```python
from build123d import *

# Parameters (mm, degrees)
BOSS_EXTRUDE1_OUTLINE_R        = 14.5
BOSS_EXTRUDE1_DEPTH            = 3.175
M4_CLEARANCE_HOLE1_D           = 4.5
F_3_3_3_3_DIAMETER_HOLE4_D     = 3.3
M3_CLEARANCE_HOLE2_D           = 3.4
M2X0_4_TAPPED_HOLE2_AT_2_COUNT = 2
M2X0_4_TAPPED_HOLE2_AT_2_PITCH = 86
M2X0_4_TAPPED_HOLE2_AT_3_COUNT = 2
M2X0_4_TAPPED_HOLE2_AT_3_PITCH = 103.730419839
M2X0_4_TAPPED_HOLE2_AT_4_COUNT = 2
M2X0_4_TAPPED_HOLE2_AT_4_PITCH = 58
FILLET1_R                      = 3
FILLET2_R                      = 1
FILLET3_SIZE                   = 6
FILLET3_SIZE_2                 = 9
FILLET4_R                      = 5
M3_CLEARANCE_HOLE1_D           = 3.4
M3_CLEARANCE_HOLE1_CSINK_D     = 3.45
M3_CLEARANCE_HOLE1_CSINK_ANGLE = 90
M2X0_4_TAPPED_HOLE1_D          = 1.6


with BuildPart() as part:
    # Boss-Extrude1: read off the stored shape, not the designer's step
    # Boss-Extrude1 outline → Boss-Extrude1 (new body)
    with BuildSketch(Plane(origin=(0, 0, 0), x_dir=(1, 0, 0), z_dir=(0, 1, 0))):
        with BuildLine():
            Line((33, 11.630595388), (33, 78.33262411))
            ThreePointArc((33, 78.33262411), (28.545123253, 80.063574355), (24, 81.541400528))
            Line((24, 81.541400528), (24, 45))
            Line((24, 45), (13, 45))
            Line((13, 45), (13, 24))
            Line((13, 24), (-13, 24))
            Line((-13, 24), (-13, 45))
            Line((-13, 45), (-24, 45))
            Line((-24, 45), (-24, 81.541400528))
            ThreePointArc((-24, 81.541400528), (-28.545123253, 80.063574355), (-33, 78.33262411))
            Line((-33, 78.33262411), (-33, 11.630595388))
            Line((-33, 11.630595388), (-49.185297029, 11.630595388))
            Line((-49.185297029, 11.630595388), (-52.624325057, 21.384301413))
            Line((-52.624325057, 21.384301413), (-58.624325057, 21.384301413))
            Line((-58.624325057, 21.384301413), (-58.624325057, 26.630595388))
            Line((-58.624325057, 26.630595388), (-68.191318528, 26.630595388))
            Line((-68.191318528, 26.630595388), (-77.073860284, 35.841596796))
            ThreePointArc((-77.073860284, 35.841596796), (-84.367778143, 10.347850562), (-83.451078309, -16.152941807))
            Line((-83.451078309, -16.152941807), (-75.073268231, -10.906716078))
            Line((-75.073268231, -10.906716078), (-66.121429656, -10.906716078))
            Line((-66.121429656, -10.906716078), (-53.091566877, -24.906716078))
            Line((-53.091566877, -24.906716078), (-34.205297029, -24.906716078))
            Line((-34.205297029, -24.906716078), (-34.205297029, -39))
            Line((-34.205297029, -39), (60.196181169, -39))
            Line((60.196181169, -39), (60.196181169, -17.27312839))
            Line((60.196181169, -17.27312839), (66.121429656, -10.906716078))
            Line((66.121429656, -10.906716078), (75.073268231, -10.906716078))
            Line((75.073268231, -10.906716078), (83.451078309, -16.152941807))
            ThreePointArc((83.451078309, -16.152941807), (84.367778143, 10.347850562), (77.073860284, 35.841596796))
            Line((77.073860284, 35.841596796), (55.268726082, 28.884301413))
            Line((55.268726082, 28.884301413), (49.185297029, 11.630595388))
            Line((49.185297029, 11.630595388), (33, 11.630595388))
        make_face()
        with Locations((-68.685297029, 8.424)):
            Circle(BOSS_EXTRUDE1_OUTLINE_R, mode=Mode.SUBTRACT)
        Polygon((-49.185297029, -18.906716078), (-49.185297029, 7.630595388), (-29, 7.630595388), (-29, 20.630595388), (-21.3, 20.630595388), (-21.3, -18.906716078), align=None, mode=Mode.SUBTRACT)
        Polygon((29, 20.630595388), (29, 7.630595388), (49.185297029, 7.630595388), (49.185297029, -27.138060345), (21.3, -27.138060345), (21.3, 20.630595388), align=None, mode=Mode.SUBTRACT)
        with Locations((68.685297029, 8.424)):
            Circle(BOSS_EXTRUDE1_OUTLINE_R, mode=Mode.SUBTRACT)
    extrude(amount=BOSS_EXTRUDE1_DEPTH)

    # M4 Clearance Hole1 (through all)
    with Locations(Plane(origin=(0, 3.175, 0), x_dir=(1, 0, 0), z_dir=(0, 1, 0))):
        with Locations((-78.54120923, -8.5016735), (78.54120923, -8.5016735)):
            Hole(M4_CLEARANCE_HOLE1_D / 2)

    # Ø3.3 (3.3) Diameter Hole4 (through all)
    with Locations(Plane(origin=(0, 3.175, 0), x_dir=(1, 0, 0), z_dir=(0, 1, 0))):
        with Locations((17.5, 15.4), (-17.5, -18), (-17.5, 15.4), (17.5, -18)):
            Hole(F_3_3_3_3_DIAMETER_HOLE4_D / 2)

    # M3 Clearance Hole2 (through all)
    with Locations(Plane(origin=(0, 3.175, 0), x_dir=(1, 0, 0), z_dir=(0, 1, 0))):
        with Locations((28.19, 74.751400528), (-28.19, 74.751400528)):
            Hole(M3_CLEARANCE_HOLE2_D / 2)

    # Sketch15 → M2x0.4 Tapped Hole2 (revolve, cut)
    with BuildSketch(Plane(origin=(-29.558455866, 3.175, -25.380595388), x_dir=(0, 0, 1), z_dir=(1, 0, 0))):
        Polygon((0, 0), (0, 3.175), (1.5, 3.175), (0.8, 2.475), (0.8, 0), align=None)
    m2x0_4_tapped_hole2 = revolve(axis=Axis((-29.558455866, 9.525, -25.380595388), (0, -1, 0)), mode=Mode.SUBTRACT)

    # M2x0.4 Tapped Hole2 at 2: M2x0.4 Tapped Hole2 ×2
    with Locations(*[(i * M2X0_4_TAPPED_HOLE2_AT_2_PITCH, 0, 0) for i in range(1, M2X0_4_TAPPED_HOLE2_AT_2_COUNT)]):
        add(m2x0_4_tapped_hole2, mode=Mode.SUBTRACT)

    # M2x0.4 Tapped Hole2 at 3: M2x0.4 Tapped Hole2 ×2
    with Locations(*[Vector(0.8290721288256765, 0, 0.5591416682777818) * (i * M2X0_4_TAPPED_HOLE2_AT_3_PITCH) for i in range(1, M2X0_4_TAPPED_HOLE2_AT_3_COUNT)]):
        add(m2x0_4_tapped_hole2, mode=Mode.SUBTRACT)

    # M2x0.4 Tapped Hole2 at 4: M2x0.4 Tapped Hole2 ×2
    with Locations(*[(0, 0, i * M2X0_4_TAPPED_HOLE2_AT_4_PITCH) for i in range(1, M2X0_4_TAPPED_HOLE2_AT_4_COUNT)]):
        add(m2x0_4_tapped_hole2, mode=Mode.SUBTRACT)

    # Fillet1
    fillet1_edges = [part.edges().sort_by_distance(p)[0] for p in [
        (75.073268231, 1.5875, 10.906716078),
        (66.121429656, 1.5875, 10.906716078),
        (-66.121429656, 1.5875, 10.906716078),
        (-75.073268231, 1.5875, 10.906716078),
        (-68.191318528, 1.5875, -26.630595388),
        (-33, 1.5875, -78.33262411),
        (-24, 1.5875, -81.541400528),
        (24, 1.5875, -81.541400528),
        (33, 1.5875, -78.33262411),
    ]]
    fillet(fillet1_edges, radius=FILLET1_R)

    # Fillet2
    fillet2_edges = [part.edges().sort_by_distance(p)[0] for p in [
        (33, 1.5875, -11.630595388),
        (49.185297029, 1.5875, -11.630595388),
        (55.268726082, 1.5875, -28.884301413),
        (77.073860284, 1.5875, -35.841596796),
        (83.451078309, 1.5875, 16.152941807),
        (60.196181169, 1.5875, 17.27312839),
        (60.196181169, 1.5875, 39),
        (-34.205297029, 1.5875, 39),
        (-34.205297029, 1.5875, 24.906716078),
        (-53.091566877, 1.5875, 24.906716078),
        (-83.451078309, 1.5875, 16.152941807),
        (-77.073860284, 1.5875, -35.841596796),
        (-58.624325057, 1.5875, -26.630595388),
        (-58.624325057, 1.5875, -21.384301413),
        (-52.624325057, 1.5875, -21.384301413),
        (-49.185297029, 1.5875, -11.630595388),
        (-33, 1.5875, -11.630595388),
        (-24, 1.5875, -45),
        (-13, 1.5875, -45),
        (13, 1.5875, -45),
        (24, 1.5875, -45),
        (-49.185297029, 1.5875, -7.630595388),
        (-21.3, 1.5875, -20.630595388),
        (-29, 1.5875, -20.630595388),
        (-29, 1.5875, -7.630595388),
        (29, 1.5875, -20.630595388),
        (21.3, 1.5875, -20.630595388),
        (49.185297029, 1.5875, -7.630595388),
        (29, 1.5875, -7.630595388),
    ]]
    fillet(fillet2_edges, radius=FILLET2_R)

    # Fillet3
    # a fillet whose section is not a circle: 9, 6 mm, written as the material it adds along each edge
    with BuildSketch(Plane(origin=(13, 0, -24), x_dir=(0, 0, -1), z_dir=(0, 1, 0))) as fillet3_piece_1:
        with BuildLine():
            Bezier((FILLET3_SIZE, 0), (0, 0), (0, FILLET3_SIZE_2), weights=[1, 0.666666667, 1])
            Line((0, FILLET3_SIZE_2), (0, 0))
            Line((0, 0), (FILLET3_SIZE, 0))
        make_face()
    extrude(amount=3.175)
    with BuildSketch(Plane(origin=(-13, 0, -24), x_dir=(1, 0, 0), z_dir=(0, 1, 0))) as fillet3_piece_2:
        with BuildLine():
            Bezier((FILLET3_SIZE_2, 0), (0, 0), (0, FILLET3_SIZE), weights=[1, 0.666666667, 1])
            Line((0, FILLET3_SIZE), (0, 0))
            Line((0, 0), (FILLET3_SIZE_2, 0))
        make_face()
    extrude(amount=3.175)

    # Fillet4
    fillet4_edges = [part.edges().sort_by_distance(p)[0] for p in [
        (-49.185297029, 1.5875, 18.906716078),
        (-21.3, 1.5875, 18.906716078),
        (21.3, 1.5875, 27.138060345),
        (49.185297029, 1.5875, 27.138060345),
    ]]
    fillet(fillet4_edges, radius=FILLET4_R)

    # M3 Clearance Hole1 (through all)
    with Locations(Plane(origin=(0, 3.175, 0), x_dir=(1, 0, 0), z_dir=(0, 1, 0))):
        with Locations((75, 29), (-75, 29)):
            CounterSinkHole(M3_CLEARANCE_HOLE1_D / 2, M3_CLEARANCE_HOLE1_CSINK_D / 2, counter_sink_angle=M3_CLEARANCE_HOLE1_CSINK_ANGLE)

    # M2x0.4 Tapped Hole1 (through all)
    with Locations(Plane(origin=(0, 3.175, 0), x_dir=(1, 0, 0), z_dir=(0, 1, 0))):
        with Locations((-20, -32), (20, -32)):
            Hole(M2X0_4_TAPPED_HOLE1_D / 2)


solid = part.part
```
Read the model definition and answer for the solid it produces. Units are mm, in the model's axes. A direction names the side the tool comes from. Round coordinates to 2 decimals unless told otherwise and drop trailing zeros. Write each loop counter-clockwise with the first axis right and the second up, starting at its lowest first coordinate (ties: lowest second). Pieces come first, ordered by that corner, then holes. Notation, with made-up numbers: (-11.5, 47) -> (0.5, 47) arc R15 ccw to (0.5, 69) -> close; hole circle Ø8 at (35, -29). An arc over 180 degrees is marked (long way). Answer in a Markdown table with one row per item. Add a question column.
1) Consider line 1 (X direction, y = 2.75, z = -46); line 2 (X direction, y = 0.25, z = 14); line 3 (Z direction, x = -69.5, y = 2.45). Determine where each line is inside the solid, lowest interval first.
2) Given P1, Ø1.5, axis at x = -67.5, y = 1, coming from the +Z side; P2, Ø1, axis at x = -70.5, y = 2.5, coming from the +Z side; P3, Ø1.6, axis at y = 1.5, z = -40.5, coming from the -X side; P4, Ø2, axis at x = -28.19, z = -74.75, coming from the +Y side (1 decimal), each flat-ended and moving along its own axis, determine where each tip first touches the part or whether it passes through.
3) Find section D-D, the plane y = 2.45. State how many separate pieces and enclosed holes the cut face has, and give its area (3 significant figures).
4) Determine the mould class of faces 5 (the face through (-24, 2, -61)), 6 (the face through (82.516, 1.565, -12.779)), 7 (the face through (-25.23, 1.61, -79.85)) for opening direction Z: pulls with the +Z half, pulls with the -Z half, needs draft (parallel to the pull), parting line crosses it, or undercut.
5) Which of the six approach directions +Z, -Z, +X, -X, +Y, -Y give full straight-line access (tool end or side, diameter ignored) to faces 1 (the face through (-79.049, 1.565, 13.396)), 2 (the face through (-35, 2, 18.907)), 3 (the face through (-84.324, 1.565, -10.697)), 4 (the face through (-50.884, 1.565, -16.449))?
6) Find section C-C, the plane x = -2. Determine the outline of the cut face in (y, z) (3 decimals), and give its area (3 significant figures).
7) Find section B-B, the plane z = -38. Determine the outline of the cut face in (x, y) (3 decimals), and give its area (3 significant figures).
8) Find section A-A, the plane x = 41. Determine the outline of the cut face in (y, z) (3 decimals), and give its area (3 significant figures).
Findings below:
| question | item | result |
|---|---|---|
| 1 | line 1 | -33 to -24, 24 to 33 |
| 1 | line 2 | -83.84 to -80.01, -63.24 to -49.18, -21.3 to 21.3, 49.19 to 63.24, 80.01 to 83.84 |
| 1 | line 3 | -27.99 to -22.9, 6.05 to 10.91 |
| 2 | P1 | z = 10.98 |
| 2 | P2 | z = 10.91 |
| 2 | P3 | x = -33 |
| 2 | P4 | through |
| 3 | separate pieces | 1 |
| 3 | enclosed holes | 20 |
| 3 | area | 6,980 mm² |
| 4 | face 5 | needs draft |
| 4 | face 6 | undercut |
| 4 | face 7 | pulls with the -Z half |
| 5 | face 1 | +Z, +Y, -Y |
| 5 | face 2 | +Y, -Y |
| 5 | face 3 | -X, +Y, -Y |
| 5 | face 4 | -Z, +Y, -Y |
| 6 | outline | (0, -24) -> (3.175, -24) -> (3.175, 39) -> (0, 39) -> close |
| 6 | area | 200 mm² |
| 7 | outline | (-33, 0) -> (-13, 0) -> (-13, 3.175) -> (-33, 3.175) -> close; (13, 0) -> (33, 0) -> (33, 3.175) -> (13, 3.175) -> close |
| 7 | area | 127 mm² |
| 8 | outline | (0, -11.631) -> (3.175, -11.631) -> (3.175, -7.631) -> (0, -7.631) -> close; (0, 27.138) -> (3.175, 27.138) -> (3.175, 39) -> (0, 39) -> close |
| 8 | area | 50.4 mm² |
